from build123d import *

# Parameters (mm, degrees)
SKETCH_1_R           = 1.625
EXTRUDE_1_DEPTH      = 4
SKETCH_2_W           = 30
SKETCH_2_H           = 11
EXTRUDE_2_DEPTH      = 4
SKETCH_3_W           = 30
SKETCH_3_H           = 24
EXTRUDE_3_DEPTH      = 4
EXTRUDE_4_DEPTH      = 30
SKETCH_5_W           = 4
SKETCH_5_H           = 23.7
EXTRUDE_5_DEPTH      = 30
SKETCH_6_W           = 30.00005
SKETCH_6_H           = 54.7
SKETCH_6_R           = 5.15
EXTRUDE_6_DEPTH      = 4
CUT_EXTRUDE_1_REACH  = 108.907
SKETCH_8_RX          = 7
SKETCH_8_RY          = 6
FILLET_START         = -32
FILLET_2_DEPTH       = 6
FILLET_3_R           = 15
EXTRUDE_8_DEPTH      = 4
EXTRUDE_8_DEPTH_BACK = 4
EXTRUDE_9_DEPTH      = 4
EXTRUDE_9_DEPTH_BACK = 4


with BuildPart() as part:
    # Эскиз1 → Бобышка-Вытянуть1 (new body)
    with BuildSketch(Plane(origin=(0, 0, 0), x_dir=(1, 0, 0), z_dir=(0, 1, 0))):
        Polygon((-10, 0), (10, 0), (10, 10), (15, 10), (15, 25.3), (-15, 25.3), (-15, 10), (-10, 10), align=None)
        with Locations(Location((-6, 15, 0), (0, 0, 270))):
            Circle(SKETCH_1_R, mode=Mode.SUBTRACT)
        with Locations(Location((0, 6, 0), (0, 0, 270))):
            Circle(SKETCH_1_R, mode=Mode.SUBTRACT)
        with Locations(Location((6, 15, 0), (0, 0, 90))):
            Circle(SKETCH_1_R, mode=Mode.SUBTRACT)
    extrude(amount=EXTRUDE_1_DEPTH)

    # Эскиз2 → Бобышка-Вытянуть2 (add)
    with BuildSketch(Plane(origin=(0, 0, -25.3), x_dir=(-1, 0, 0), z_dir=(0, 0, -1))):
        with Locations((0, -1.5)):
            Rectangle(SKETCH_2_W, SKETCH_2_H)
    extrude(amount=EXTRUDE_2_DEPTH)

    # Эскиз3 → Бобышка-Вытянуть3 (add)
    with BuildSketch(Plane.XZ.offset(7)):
        with Locations((0, -37.3)):
            Rectangle(SKETCH_3_W, SKETCH_3_H)
    extrude(amount=-EXTRUDE_3_DEPTH)

    # Эскиз4 → Бобышка-Вытянуть4 (add, through all)
    with BuildSketch(Plane.ZY.offset(15)):
        Polygon((-29.3, 4), (-29.3, -3), (-49.3, -3), align=None)
    extrude(amount=-EXTRUDE_4_DEPTH)

    # Эскиз5 → Бобышка-Вытянуть5 (add, through all)
    with BuildSketch(Plane(origin=(15, 0, 0), x_dir=(0, 0, -1), z_dir=(1, 0, 0))):
        with Locations((47.3, -18.85)):
            Rectangle(SKETCH_5_W, SKETCH_5_H)
    extrude(amount=-EXTRUDE_5_DEPTH)

    # Эскиз6 → Бобышка-Вытянуть6 (add)
    with BuildSketch(Plane.XZ.offset(30.7)):
        with Locations((-2.5e-05, -72.65)):
            Rectangle(SKETCH_6_W, SKETCH_6_H)
        with Locations(Location((-2.5e-05, -84, 0), (0, 0, 270))):
            Circle(SKETCH_6_R, mode=Mode.SUBTRACT)
    extrude(amount=-EXTRUDE_6_DEPTH)

    # Эскиз8 → Вырез-Вытянуть1 (cut, up to next)
    with BuildSketch(Plane.XZ.offset(30.7), mode=Mode.PRIVATE) as cut_extrude_1_sk1:
        with Locations(Location((15, -65.3), (0, 0, -90))):
            Ellipse(SKETCH_8_RX, SKETCH_8_RY)
    cut_extrude_1_tool1 = extrude(cut_extrude_1_sk1.sketch, amount=-CUT_EXTRUDE_1_REACH, mode=Mode.PRIVATE) & part.part
    # Эскиз8 → Вырез-Вытянуть1 (cut, up to next)
    with BuildSketch(Plane.XZ.offset(30.7), mode=Mode.PRIVATE) as cut_extrude_1_sk2:
        with Locations(Location((-15.000018282, -65.299986289), (0, 0, -90.000052373))):
            Ellipse(SKETCH_8_RX, SKETCH_8_RY)
    cut_extrude_1_tool2 = extrude(cut_extrude_1_sk2.sketch, amount=-CUT_EXTRUDE_1_REACH, mode=Mode.PRIVATE) & part.part
    add(cut_extrude_1_tool1.solids().sort_by_distance((15, -30.7, -65.3))[0], mode=Mode.SUBTRACT)
    add(cut_extrude_1_tool2.solids().sort_by_distance((-15.000018, -30.7, -65.299986))[0], mode=Mode.SUBTRACT)

    # Скругление2: read off the stored shape, not the designer's step
    # Скругление2 outline → Скругление2 (cut)
    with BuildSketch(Plane(origin=(0, 0, 0), x_dir=(1, 0, 0), z_dir=(0, 1, 0)).offset(FILLET_START)):
        with BuildLine():
            Line((15, 72.3), (15, 73.218180859))
            ThreePointArc((15, 73.218180859), (14.762336304, 72.570999772), (14.162313281, 72.231441583))
            add(Edge.make_bspline(
                [(14.162313281, 72.231441583), (14.579095458, 72.3), (15, 72.3)],
                knots=[6.131749827, 6.131749827, 6.131749827, 6.283185307, 6.283185307, 6.283185307], degree=2, weights=[0.948970652, 0.971763096, 1]))
        make_face()
        with BuildLine():
            add(Edge.make_bspline(
                [(15, 58.3), (14.579095458, 58.3), (14.162313281, 58.368558417)],
                knots=[3.141592654, 3.141592654, 3.141592654, 3.293028134, 3.293028134, 3.293028134], degree=2, weights=[1, 0.971763096, 0.948970652]))
            ThreePointArc((14.162313281, 58.368558417), (14.762336304, 58.029000228), (15, 57.381819141))
            Line((15, 57.381819141), (15, 58.3))
        make_face()
        with BuildLine():
            add(Edge.make_bspline(
                [(-15.00005, 72.299986289), (-14.579143154, 72.299988746), (-14.162358429, 72.231432015)],
                knots=[6.283181087, 6.283181087, 6.283181087, 6.434617466, 6.434617466, 6.434617466], degree=2, weights=[1, 0.971762843, 0.948970209]))
            ThreePointArc((-14.162358429, 72.231432015), (-14.762384713, 72.570989127), (-15.00005, 73.218172089))
            Line((-15.00005, 73.218172089), (-15.00005, 72.299986289))
        make_face()
        with BuildLine():
            ThreePointArc((-15.00005, 57.381799936), (-14.762384538, 58.028983103), (-14.162357897, 58.368540098))
            add(Edge.make_bspline(
                [(-14.162357897, 58.368540098), (-14.579142884, 58.299983554), (-15.00005, 58.299986289)],
                knots=[9.27334784, 9.27334784, 9.27334784, 9.424784314, 9.424784314, 9.424784314], degree=2, weights=[0.948970181, 0.971762826, 1]))
            Line((-15.00005, 58.299986289), (-15.00005, 57.381799936))
        make_face()
    extrude(amount=FILLET_2_DEPTH, mode=Mode.SUBTRACT)

    # Скругление3
    fillet_3_edges = [part.edges().sort_by_distance(p)[0] for p in [
        (-15.00005, -28.7, -100),
        (15, -28.7, -100),
    ]]
    fillet(fillet_3_edges, radius=FILLET_3_R)

    # Эскиз10 → Бобышка-Вытянуть8 (add, two sides: drawn at the far end of the back side and taken through both)
    with BuildSketch(Plane.ZY.offset(2.5e-05).offset(-EXTRUDE_8_DEPTH_BACK)):
        Polygon((-49.3, -26.7), (-73.3, -26.7), (-49.3, -3), align=None)
    extrude(amount=EXTRUDE_8_DEPTH + EXTRUDE_8_DEPTH_BACK)

    # Эскиз11 → Бобышка-Вытянуть9 (add, two sides: drawn at the far end of the back side and taken through both)
    with BuildSketch(Plane.ZY.offset(2.5e-05).offset(-EXTRUDE_9_DEPTH_BACK)):
        Polygon((-31.3, -7), (-45.3, -7), (-45.3, -30.7), align=None)
    extrude(amount=EXTRUDE_9_DEPTH + EXTRUDE_9_DEPTH_BACK)


solid = part.part
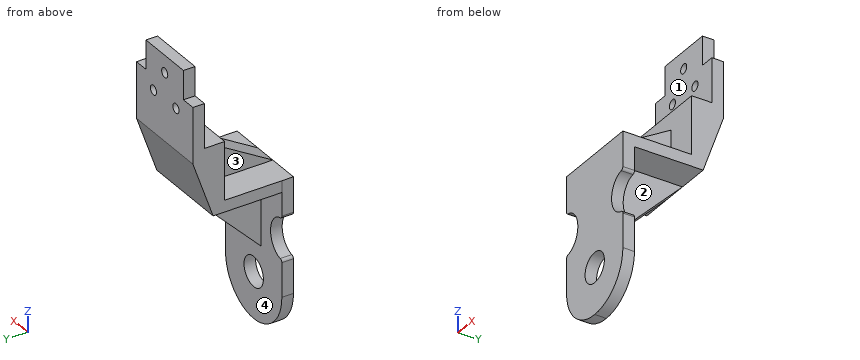
Can you work these out from the model? Positions are in its coordinate system, mm. Face numbers are marked on the shaded views. A direction names the side the tool comes from. Coordinates: 2 decimals unless noted, no trailing zeros. Write each loop counter-clockwise with the first axis right and the second up, starting at its lowest first coordinate (ties: lowest second). Pieces come first, ordered by that corner, then holes.
Q1. Imagine slicing it at D-D, the plane y = 1. List the corners of the cut face in (x, z) for me (3 decimals), plus the area to 3 significant figures.
Results found:
outline: (-15, -37.871) - (15, -37.871) - (15, -10) - (10, -10) - (10, 0) - (-10, 0) - (-10, -10) - (-15, -10) - close; hole circle Ø3.25 at (-6, -15); hole circle Ø3.25 at (0, -6); hole circle Ø3.25 at (6, -15)
area: 1,010 mm2
Q2. Imagine slicing it at A-A, the plane z = -15. List the corners of the cut face in (x, y) for me (3 decimals).
Results found:
outline: (-15, 0) - (-7.625, 0) - (-7.625, 4) - (-15, 4) - close; (-4.375, 0) - (4.375, 0) - (4.375, 4) - (-4.375, 4) - close; (7.625, 0) - (15, 0) - (15, 4) - (7.625, 4) - close
Q3. Imagine slicing it at C-C, the plane x = 3. List the corners of the cut face in (y, z) for me.
Results found:
outline: (-30.7, -99.7) - (-26.7, -99.7) - (-26.7, -88.19) - (-30.7, -88.19) - close; (-30.7, -79.81) - (-26.7, -79.81) - (-26.7, -73.3) - (-3, -49.3) - (4, -29.3) - (4, 0) - (0, 0) - (0, -25.3) - (-7, -25.3) - (-7, -31.3) - (-30.7, -45.3) - close
Q4. Imagine slicing it at B-B, the plane z = -84. List the corners of the cut face in (x, y) for me.
Results found:
outline: (-15, -30.7) - (-5.15, -30.7) - (-5.15, -26.7) - (-15, -26.7) - close; (5.15, -30.7) - (15, -30.7) - (15, -26.7) - (5.15, -26.7) - close
Q5. Which directions (+Z, -Z, +X, -X, +Y, -Y) give clear straight access to the entire face, cutting with the end or side of a thin tool? Please do the marked faces 1, 2, 3 and 4.
Results found:
face 1: +Z, +X, -X, -Y
face 2: -Z, +X, +Y
face 3: +Z, -X, -Y
face 4: -Z, +Y
Q6. For P1, Ø2, axis at x = -6, z = -11, coming from the -Y side; P2, Ø10, axis at x = 1, z = -36, coming from the -Y side; P3, Ø3.5, axis at x = 12, y = -19.5, coming from the -Z side; P4, Ø5, axis at x = -6, z = -15, coming from the +Y side, each with a flat end and sliding along its axis, tell me the tip position at first contact or that it passes through.
Results found:
P1: stops at y = 0
P2: stops at y = -23.42
P3: stops at z = -49.3
P4: stops at y = 4
Q7. Please list where these lines run through material, in increasing order: L1, parallel to X at y = 2, z = -15 (3 decimals); L2, parallel to X at y = -29.8, z = -84; L3, parallel to X at y = 2, z = -6 (3 decimals).
Results found:
L1: x = -15 to -7.625, -4.375 to 4.375, 7.625 to 15
L2: x = -15 to -5.15, 5.15 to 15
L3: x = -10 to -1.625, 1.625 to 10
